Here's how the part is built. I have some questions about the finished solid (model axes, mm). A direction names the side the tool comes from. Round coordinates to 2 decimals unless told otherwise and drop trailing zeros. Write each loop counter-clockwise with the first axis right and the second up, starting at its lowest first coordinate (ties: lowest second). Pieces come first, ordered by that corner, then holes. Notation, with made-up numbers: (-27, 55.25) -> (-5, 55.25) arc R22 ccw to (-5, 85.25) -> close; hole circle Ø2 at (61.25, 13). An arc over 180 degrees is marked (long way). Put each result on its own line as item: value. Start each with the question number.
1) I want a section at A-A, the plane x = -27.5. List the corners of the cut face in (y, z) for me.
2) I want a section at D-D, the plane y = -8.5. List the corners of the cut face in (x, z) for me.
3) I want a section at B-B, the plane y = 47.5. List the corners of the cut face in (x, z) for me.
4) If I drill on line 1 along X through (y, z) = (28, -3.5); line 2 along Y through (x, z) = (-32, -6.5); line 3 along Z through (x, y) = (-16, -3), over which ranges is the centre line in solid material (lowest first)? Write a range as [from, to].
5) We'd pull the mould along X, two halves only. Please class faces 6 (the cylindrical face through (-4.17, 60.96, -4.93)), 7 (the flat face through (-21, 4, 2)), 8 (the cylindrical face through (-8.79, 59.356, -3.916)): released by +X, released by -X, zero draft, split by the parting line, or undercut.
6) Will these pins go through, and if not, where does the flat tip stop? P1, Ø1, axis at x = 14.5, z = -6.5, coming from the -Y side; P2, Ø3, axis at x = -13.5, z = -7.5, coming from the -Y side; P3, Ø12, axis at x = -4, y = -29.5, coming from the +Z side.
7) Which directions (+Z, -Z, +X, -X, +Y, -Y) give clear straight access to the entire face, cutting with the end or side of a thin tool? Please do faces 1 (the flat face through (-6.45, -3.63, -4.93)), 2 (the flat face through (-4, -33, 0)), 3 (the flat face through (-5, -3, -10)), 4 (the flat face through (-18.1, 1, 0)), 5 (the flat face through (-7.437, -27.783, -4.93)).
8) I want a section at C-C, the plane z = -8.25. List the corners of the cut face in (x, y) for me.
from build123d import *

# Parameters (mm, degrees)
F1_DEPTH = 10
F2_R     = 31.347396
F3_DEPTH = 10
F4_R     = 35.277865
F5_DEPTH = 2
F6_R     = 29.989336
F7_DEPTH = 25


with BuildPart() as f1:
    # F0 (on Top) → F1 (new body)
    with BuildSketch(Plane.XY):
        Polygon((0, 0), (-10.077596, 0), (-4.275343, -5.802252), (-10.688359, -50.387979), (0, -50.387979), align=None)
    extrude(amount=-F1_DEPTH)

    # F2 (on Top) → F3 (join)
    with BuildSketch(Plane.XY):
        with Locations((-4.886107, 29.622024)):
            Circle(F2_R)
    extrude(amount=-F3_DEPTH)

    # F4 (on face) → F5 (join)
    with BuildSketch(Plane.XY):
        with Locations((-4.886107, 29.622024)):
            Circle(F4_R)
    extrude(amount=F5_DEPTH)

    # F6 (on face) → F7 (cut)
    with BuildSketch(Plane.XY.offset(2)):
        with Locations((-4.886107, 29.622024)):
            Circle(F6_R)
    extrude(amount=-F7_DEPTH, mode=Mode.SUBTRACT)


solid = f1.part
Findings:
1. outline: (2.55, 0) -> (7.91, 0) -> (7.91, -10) -> (9.93, -10) -> (9.93, 2) -> (2.55, 2) -> close; (49.32, -10) -> (51.33, -10) -> (51.33, 0) -> (56.7, 0) -> (56.7, 2) -> (49.32, 2) -> close
2. outline: (-4.66, -10) -> (0, -10) -> (0, 0) -> (-4.66, 0) -> close
3. outline: (-35.3, 0) -> (-30.64, 0) -> (-30.64, -10) -> (-28.96, -10) -> (-28.96, 2) -> (-35.3, 2) -> close; (19.19, -10) -> (20.86, -10) -> (20.86, 0) -> (25.53, 0) -> (25.53, 2) -> (19.19, 2) -> close
4. line 1: x = [-36.19, -34.83], [25.06, 26.42]
4. line 2: y = [13.89, 16.81], [42.44, 45.35]
4. line 3: z = [0, 2]
5. face 6: split by the parting line
5. face 7: zero draft
5. face 8: undercut
6. P1: stops at y = 4.6
6. P2: stops at y = -0.91
6. P3: stops at z = 0
7. face 1: -Z, -X
7. face 2: +Z, +X, -X, -Y
7. face 3: -Z, +X, -X, +Y, -Y
7. face 4: -Z
7. face 5: +Z, -Z, -X
8. outline: (-10.69, -50.39) -> (0, -50.39) -> (0, -1.34) arc R31.35 ccw (long way) to (-8.57, -1.51) -> (-4.28, -5.8) -> close; hole circle Ø59.98 at (-4.89, 29.62)
